Verification items for the finished model (mm, model axes). Round coordinates to 2 decimals unless told otherwise and drop trailing zeros. Loops run counter-clockwise (first coordinate to the right, second up) from the corner with the lowest first, then second, coordinate; pieces in that order, holes last.
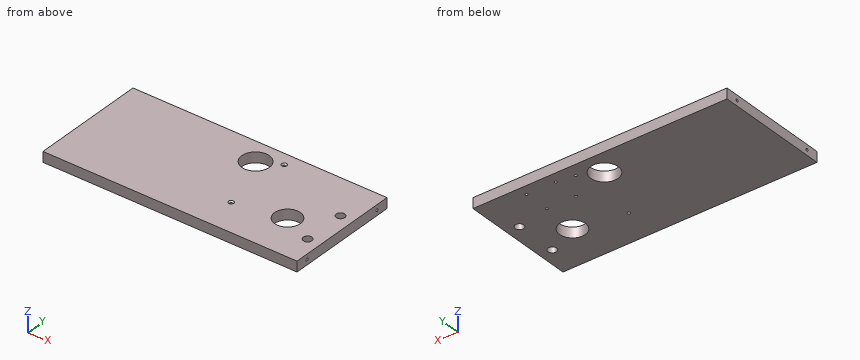
from build123d import *

# Parameters (mm, degrees)
SKETCH1_W           = 296
SKETCH1_H           = 134
SKETCH1_R           = 15
SKETCH1_R_2         = 16
SKETCH1_R_3         = 5
SKETCH1_R_4         = 1.5
BOSS_EXTRUDE1_DEPTH = 12
CUT_EXTRUDE1_START  = 12.189127
SKETCH2_R           = 1.5
CUT_EXTRUDE1_DEPTH  = 20
CUT_EXTRUDE2_START  = 288.189127
SKETCH2_2_R         = 1.5
CUT_EXTRUDE2_DEPTH  = 20.000001
SKETCH5_R           = 1.5
CUT_EXTRUDE5_DEPTH  = 10


with BuildPart() as part:
    # Sketch1 → Boss-Extrude1 (new body)
    with BuildSketch(Plane.XY):
        with Locations((160.18912744, 67)):
            Rectangle(SKETCH1_W, SKETCH1_H)
        with Locations((257.18912744, 51)):
            Circle(SKETCH1_R, mode=Mode.SUBTRACT)
        with Locations((176.18912744, 107)):
            Circle(SKETCH1_R_2, mode=Mode.SUBTRACT)
        with Locations((293.18912744, 84)):
            Circle(SKETCH1_R_3, mode=Mode.SUBTRACT)
        with Locations((200.18912744, 119)):
            Circle(SKETCH1_R_4, mode=Mode.SUBTRACT)
        with Locations((200.18912744, 40)):
            Circle(SKETCH1_R_4, mode=Mode.SUBTRACT)
        with Locations((293.18912744, 35)):
            Circle(SKETCH1_R_3, mode=Mode.SUBTRACT)
    extrude(amount=BOSS_EXTRUDE1_DEPTH)

    # Sketch2 → Cut-Extrude1 (cut)
    with BuildSketch(Plane(origin=(0, 0, 0), x_dir=(0, 0, -1), z_dir=(1, 0, 0)).offset(CUT_EXTRUDE1_START)):
        with Locations((-6, 119)):
            Circle(SKETCH2_R)
        with Locations((-6, 15)):
            Circle(SKETCH2_R)
    extrude(amount=CUT_EXTRUDE1_DEPTH, mode=Mode.SUBTRACT)

    # Sketch2<2> → Cut-Extrude2 (cut)
    with BuildSketch(Plane(origin=(0, 0, 0), x_dir=(0, 0, -1), z_dir=(1, 0, 0)).offset(CUT_EXTRUDE2_START)):
        with Locations((-6, 119)):
            Circle(SKETCH2_2_R)
        with Locations((-6, 15)):
            Circle(SKETCH2_2_R)
    extrude(amount=CUT_EXTRUDE2_DEPTH, mode=Mode.SUBTRACT)

    # Cut-Extrude4 cone 1 section (through the dimple's axis) → Cut-Extrude4 (revolve, cut)
    with BuildSketch(Plane(origin=(200.18912744, 119, 12), x_dir=(0, -1, 0), z_dir=(1, 0, 0))):
        Polygon((0, 0), (3, 0), (0, 3), align=None)
    revolve(axis=Axis((200.18912744, 119, 12), (0, 0, -1)), mode=Mode.SUBTRACT)

    # Cut-Extrude4 cone 2 section (through the dimple's axis) → Cut-Extrude4 cone 2 (revolve, cut)
    with BuildSketch(Plane(origin=(200.18912744, 40, 12), x_dir=(0, -1, 0), z_dir=(1, 0, 0))):
        Polygon((0, 0), (3, 0), (0, 3), align=None)
    revolve(axis=Axis((200.18912744, 40, 12), (0, 0, -1)), mode=Mode.SUBTRACT)

    # Sketch5 → Cut-Extrude5 (cut)
    with BuildSketch(Plane.XY):
        with Locations(Location((221.18912744, 122, 0), (0, 0, 180))):
            Circle(SKETCH5_R)
        with Locations(Location((255.18912744, 122, 0), (0, 0, 180))):
            Circle(SKETCH5_R)
        with Locations(Location((221.18912744, 92, 0), (0, 0, 180))):
            Circle(SKETCH5_R)
        with Locations(Location((255.18912744, 92, 0), (0, 0, 180))):
            Circle(SKETCH5_R)
    extrude(amount=CUT_EXTRUDE5_DEPTH, mode=Mode.SUBTRACT)


solid = part.part
1. Scan lines: L1, parallel to X at y = 109.5, z = 9.75; L2, parallel to X at y = 49.5, z = 4. Record each from-to range of solid material in increasing order.
2. Gauge pin test, flat ends, axial feed: P1, Ø1.8, axis at y = 119, z = 6, coming from the -X side; P2, Ø1.8, axis at x = 200.19, y = 40, coming from the +Z side; P3, Ø0.9, axis at x = 221, y = 121.5, coming from the -Z side. Record the tip position at first contact, or that the pin passes through.
3. Section check C-C (y = 47). Enter the section's corners in (x, z).
4. Section check A-A (z = 2.25). Give the number of separate pieces and of enclosed holes in the cut face, then the cut area to 3 significant figures.
5. Section check B-B (y = 84). Enter the section's corners in (x, z).
Taken from the geometry:
1. L1: x = 12.19 to 160.39, 191.99 to 308.19
1. L2: x = 12.19 to 242.26, 272.11 to 308.19
2. P1: stops at x = 32.19
2. P2: passes through
2. P3: stops at z = 10
3. outline: (12.19, 0) - (242.73, 0) - (242.73, 12) - (12.19, 12) - close; (271.65, 0) - (308.19, 0) - (308.19, 12) - (271.65, 12) - close
4. separate pieces: 1
4. enclosed holes: 10
4. area: 38,000 mm2
5. outline: (12.19, 0) - (288.19, 0) - (288.19, 12) - (12.19, 12) - close; (298.19, 0) - (308.19, 0) - (308.19, 12) - (298.19, 12) - close
